Autodesk Inventor part; units mm, degrees
ref_plane "Work Plane2" through (0, 125, 0) normal (0, 1, 0) x (-1, 0, 0)
ref_plane "Work Plane3" through (43, 0, 0) normal (1, 0, 0) x (0, 1, 0)
ref_plane "Work Plane4" through (0, 0, 43) normal (0, 0, 1) x (1, 0, 0)
sketch "Sketch3" plane through (0, 0, 0) normal (0, 1, 0) x (-1, 0, 0)
  circle A0 centre (0, 0) radius 43
  circle A1 centre (0, 0) radius 42
  dimension "d8" = 86
  dimension "d9" = 84
extrude "Extrusion3" add sketch "Sketch3" along normal blind 250
ref_plane "Work Plane2" through (0, 125, 0) normal (0, 1, 0) x (-1, 0, 0)
sketch "Sketch4" plane through (0, 250, 0) normal (0, 1, 0) x (1, 0, 0)
  circle A0 centre (0, 42.5) radius 0.25
  point P0 (0, 0)
  dimension "d12" = 0.5
  dimension "d13" = 42.5
extrude "Extrusion4" cut sketch "Sketch4" along normal through all both and the other way through all
mirror "Mirror1" about plane through (0, 0, 0) normal (0, 0, 1) of "Extrusion4"
ref_plane "Work Plane3" through (43, 0, 0) normal (1, 0, 0) x (0, 1, 0)
sketch "Sketch5" plane through (43, 0, 0) normal (1, 0, 0) x (0, 1, 0)
  circle A0 centre (150, 0) radius 1
  point P0 (0, 0)
  dimension "d16" = 2
extrude "Extrusion5" cut sketch "Sketch5" against normal through all
ref_plane "Work Plane4" through (0, 0, 43) normal (0, 0, 1) x (1, 0, 0)
sketch "Sketch6" plane through (0, 0, 43) normal (0, 0, 1) x (1, 0, 0)
  circle A0 centre (-0.25, 150) radius 1
  point P0 (0, 0)
extrude "Extrusion6" cut sketch "Sketch6" against normal through all
properties part number "seed_holder"
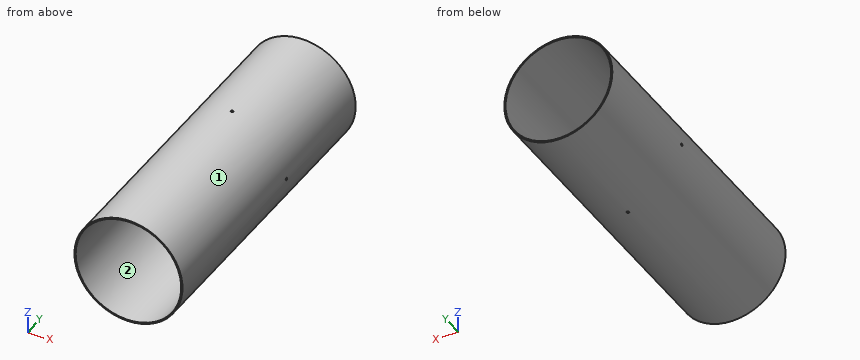
Geometry check sheet. Reference: the model listing, model coordinates, mm. Face numbers are marked on the shaded views. Give positions to 0.01 mm unless a question says otherwise; leave off trailing zeros. Loops run counter-clockwise (first coordinate to the right, second up) from the corner with the lowest first, then second, coordinate; pieces in that order, holes last. Notation, with made-up numbers: M -8.75,-3.75 L -4.75,-3.75 A13 cw -4.75,2.25 Z; hole C 45,38.5 d5. An arc over 180 degrees is marked long. Write item = value, one per line.
(1) Material ranges on line 1 (Z direction, x = 0, y = 52); line 2 (Y direction, x = -0.25, z = 42.3); line 3 (Z direction, x = 1, y = 74), recorded low to high. Write a range as [from, to].
Answer below:
line_1 = [-43, -42.75], [-42.25, -42], [42, 42.25], [42.75, 43]
line_2 = [0, 149], [151, 250]
line_3 = [-42.99, -41.99], [41.99, 42.99]
(2) Gauge pin test, flat ends, axial feed: pin 1 Ø5 at (y, z) = (144.5, -15) entering from -X; pin 2 Ø4 at (y, z) = (213, -25) entering from +X; pin 3 Ø12 at (y, z) = (166.5, 17) entering from +X; pin 4 Ø10 at (x, z) = (-32.5, 7.5) entering from +Y. Record the tip position at first contact, or that the pin passes through.
Answer below:
pin_1 = -41.14
pin_2 = 36.33
pin_3 = 41.57
pin_4 = through
(3) Sectioned sample at C-C, the plane y = 100. Record the cut outline in (x, z).
Answer below:
outline = C 0,0 d86; hole C 0,0 d84; hole C 0,-42.5 d0.5; hole C 0,42.5 d0.5
(4) Release check for a two-part mould opening along X. For the marked faces 1 and 2 record: released by +X, released by -X, zero draft, split by the parting line, or undercut.
Answer below:
face_1 = split by the parting line
face_2 = undercut
(5) Sectioned sample at A-A, the plane z = -4.5. Record the cut outline in (x, y).
Answer below:
outline = M -42.76,0 L -41.76,0 L -41.76,250 L -42.76,250 Z; M 41.76,0 L 42.76,0 L 42.76,250 L 41.76,250 Z
(6) Sectioned sample at B-B, the plane x = 4.5. Record the cut outline in (y, z), plus the area to 3 significant figures.
Answer below:
outline = M 0,-42.76 L 250,-42.76 L 250,-41.76 L 0,-41.76 Z; M 0,41.76 L 250,41.76 L 250,42.76 L 0,42.76 Z
area = 503 mm2
